from build123d import *


with BuildPart() as part:
    # Sketch1 → Revolve1 (revolve)
    with BuildSketch(Plane.XY):
        with BuildLine():
            Line((-7.1374, 6.4135), (5.721708584, 6.4135))
            Line((5.721708584, 6.4135), (7.1374, 7.4803))
            Line((7.1374, 7.4803), (7.1374, 8.2804))
            ThreePointArc((7.1374, 8.2804), (7.025807684, 8.549807684), (6.7564, 8.6614))
            Line((6.7564, 8.6614), (1.9558, 8.6614))
            ThreePointArc((1.9558, 8.6614), (1.686392316, 8.549807684), (1.5748, 8.2804))
            Line((1.5748, 8.2804), (1.5748, 7.1374))
            Line((1.5748, 7.1374), (-7.1374, 7.1374))
            Line((-7.1374, 7.1374), (-7.1374, 6.4135))
        make_face()
    revolve(axis=Axis((-7.1374, 0, 0), (1, 0, 0)))


solid = part.part
The listing builds one solid part. Answer for the finished solid, in the listing's coordinates (mm). A direction names the side the tool comes from. Give positions to 0.01 mm unless a question says otherwise; leave off trailing zeros. Order: outer loops, then holes, each group sorted by start corner. A loop starts at its lowest first (then second) coordinate and runs counter-clockwise, first axis right, second up. Notation, with made-up numbers: (46.5, 73) - (103.5, 73) arc R21 cw to (103.5, 106) - close; hole circle Ø2 at (77.25, 25). An arc over 180 degrees is marked (long way). Use one line per item in the form item = value.
1) Find section A-A on z = 0. Determine the outline of the cut face in (x, y), and give its area (3 significant figures).
Verdict:
outline = (-7.14, -7.14) - (1.57, -7.14) - (1.57, -8.28) arc R0.38 ccw to (1.96, -8.66) - (6.76, -8.66) arc R0.38 ccw to (7.14, -8.28) - (7.14, -7.48) - (5.72, -6.41) - (-7.14, -6.41) - close; (-7.14, 6.41) - (5.72, 6.41) - (7.14, 7.48) - (7.14, 8.28) arc R0.38 ccw to (6.76, 8.66) - (1.96, 8.66) arc R0.38 ccw to (1.57, 8.28) - (1.57, 7.14) - (-7.14, 7.14) - close
area = 36.0 mm^2
2) Find section C-C on x = 4.25. Determine the outline of the cut face in (y, z), and give its area (3 significant figures).
Verdict:
outline = circle Ø17.32 at (0, 0); hole circle Ø12.83 at (0, 0)
area = 106 mm^2
3) Each of these flat-tipped pins is pushed along its axis until it touches: pin 1 (2 mm diameter, centred on x = 5.5, z = -4.5, fed in from -Y); pin 2 (3 mm diameter, centred on x = -4, z = 3, fed in from +Y); pin 3 (4 mm diameter, centred on x = 5.5, z = -2.5, fed in from -Y). Where does it stop, or does it pass through?
Verdict:
pin_1 = -7.92
pin_2 = 6.98
pin_3 = -8.65
4) Find section D-D on x = -0.5. Determine the outline of the cut face in (y, z).
Verdict:
outline = circle Ø14.27 at (0, 0); hole circle Ø12.83 at (0, 0)
5) For faces 1 (the flat face through (1.575, 0, 7.4)), 2 (the flat face through (7.137, 4, -7)), determine the directions among +Z, -Z, +X, -X, +Y, -Y from which every point of the face is accessible in a straight line to the end or side of a thin tool.
Verdict:
face_1 = -X
face_2 = +Z, -Z, +X, +Y, -Y
6) Consider probe 1 along Z at (x, y) = (-3, 0); probe 2 along Z at (x, y) = (3.25, 0); probe 3 along X at (y, z) = (-3, 6.25). Determine where each line is inside the solid, lowest interval first. Write a range as [from, to].
Verdict:
probe_1 = [-7.14, -6.41], [6.41, 7.14]
probe_2 = [-8.66, -6.41], [6.41, 8.66]
probe_3 = [-7.14, 6.41]
7) The mould has two halves that part along Z. Classify faces 3 (the flat face through (-7.137, -6, 3)), 4 (the cylindrical face through (-0.618, 6.117, 1.926)), 5 (the cylindrical face through (-2.84, -7.13, 0.31)): released by +Z, released by -Z, zero draft, split by the parting line, or undercut.
Verdict:
face_3 = zero draft
face_4 = undercut
face_5 = split by the parting line
